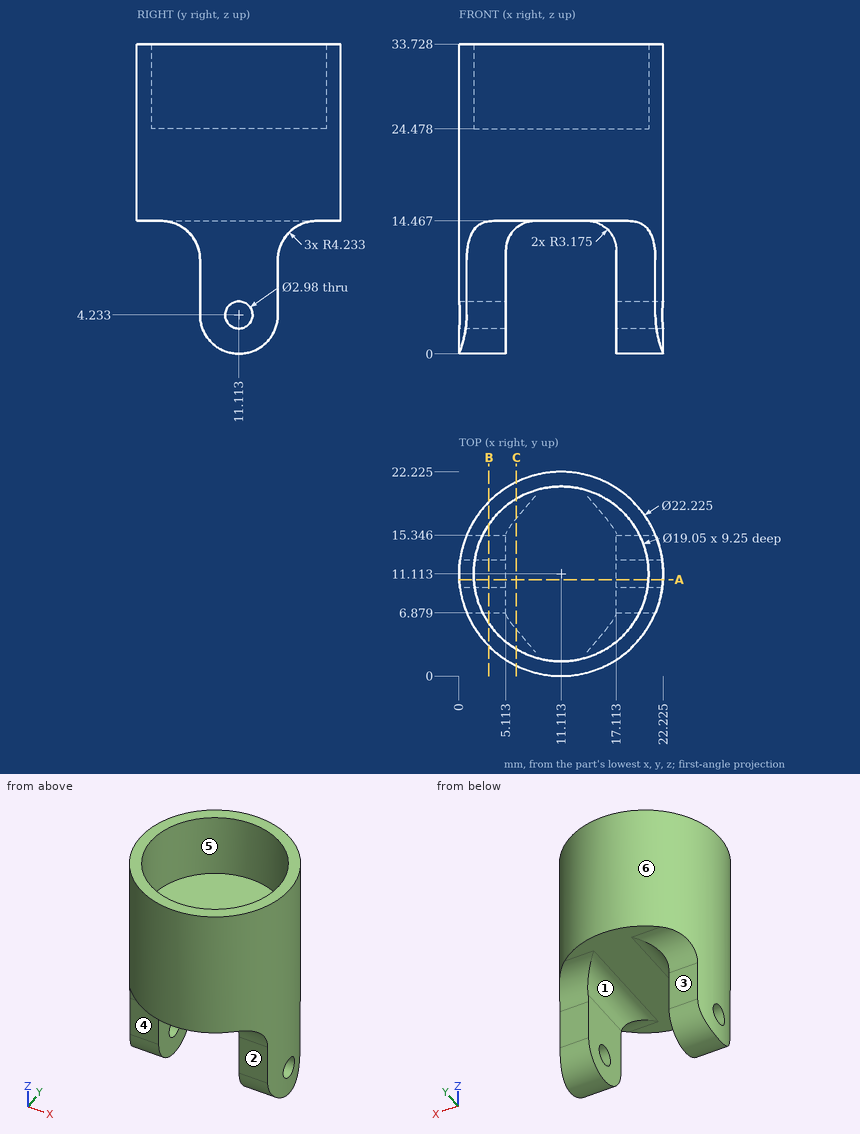
Drawing for the job (mm, zero at the part's lowest x, y, z). A direction names the side the tool comes from. Coordinates: 2 decimals unless noted, no trailing zeros. Order: outer loops, then holes, each group sorted by start corner. A loop starts at its lowest first (then second) coordinate and runs counter-clockwise, first axis right, second up. Notation, with made-up numbers: (-8.5, -12) - (34.5, -12) arc R32 ccw to (34.5, 15) - close; hole circle Ø10 at (54.5, -11.5). An arc over 180 degrees is marked (long way). Use a Markdown table: item, result. Add a question column.
(1) Pull direction X, two halves, no side cores. Call the marked faces 4, 5 and 6: +X half, -X half, draft (parallel to the pull), parting line (faces both ways), or undercut.
(2) Flat gauge pins, fed straight in: pin 1 (11.5 mm diameter, centred on x = 11.11, y = 11.11, fed in from +Z); pin 2 (8 mm diameter, centred on y = 15, z = 26.5, fed in from -X); pin 3 (1.3 mm diameter, centred on x = 19, z = 8, fed in from -Y); pin 4 (4 mm diameter, centred on x = 8.5, z = 21, fed in from -Y). Where does each tip first touch, or does it go through?
(3) Saw through at C-C (x = 6.25). Give the cut face in (y, z) (1 decimal).
(4) Which spindle directions (+Z, -Z, +X, -X, +Y, -Y) get a long thin tool onto all of the face, cutting with end or side? Do the marked faces 1, 2 and 3. Say none if no direction does.
(5) Saw through at A-A (y = 10.5). Count the separate pieces of the cut face and the enclosed holes in it, then the cut area to 3 significant figures.
(6) Saw through at B-B (x = 3.25). Give the cut face in (y, z) (1 decimal).
(7) Drill centre lines: line 1 along Z through (x, y) = (15.25, 19.5) (1 decimal); line 2 along Y through (x, z) = (17.25, 7.5) (1 decimal); line 3 along X through (y, z) = (5, 29) (1 decimal). Where is each one in solid material? Low to high. Write a range as [from, to].
Solved:
| question | item | result |
|---|---|---|
| 1 | face 4 | draft |
| 1 | face 5 | undercut |
| 1 | face 6 | parting line |
| 2 | pin 1 | stops at z = 24.48 |
| 2 | pin 2 | stops at x = 0 |
| 2 | pin 3 | stops at y = 6.88 |
| 2 | pin 4 | stops at y = 0.02 |
| 3 | outline | (1.1, 14.5) - (2.6, 14.5) arc R4.2 cw to (5, 13.7) - (17.2, 13.7) arc R4.2 cw to (19.6, 14.5) - (21.1, 14.5) - (21.1, 33.7) - (19.3, 33.7) - (19.3, 24.5) - (2.9, 24.5) - (2.9, 33.7) - (1.1, 33.7) - close |
| 4 | face 1 | -Z, +Y, -Y |
| 4 | face 2 | -Z, +X, -X, -Y |
| 4 | face 3 | -Z, +X, -X, +Y |
| 5 | separate pieces | 3 |
| 5 | enclosed holes | 0 |
| 5 | area | 375 mm² |
| 6 | outline | (3.3, 14.4) arc R4.2 cw to (6.9, 10.2) - (6.9, 4.2) arc R4.2 ccw to (15.3, 4.2) - (15.3, 10.2) arc R4.2 cw to (19, 14.4) - (19, 33.7) - (16.5, 33.7) - (16.5, 24.5) - (5.7, 24.5) - (5.7, 33.7) - (3.3, 33.7) - close; hole circle Ø3 at (11.1, 4.2) |
| 7 | line 1 | z = [14.5, 24.5] |
| 7 | line 2 | y = [6.9, 15.3] |
| 7 | line 3 | x = [1.8, 3.8], [18.4, 20.4] |
